Can you work these out from the model? Positions are in its coordinate system, mm. A direction names the side the tool comes from. Coordinates: 2 decimals unless noted, no trailing zeros. Order: outer loops, then holes, each group sorted by start corner. A loop starts at its lowest first (then second) coordinate and runs counter-clockwise, first axis right, second up. Notation, with made-up numbers: (-13, 87) -> (34, 87) arc R22 ccw to (34, 97) -> close; hole circle Ø7 at (-27.75, -11). An arc over 180 degrees is marked (long way). Return JSON: item names as keys, results as strings. Group by question number.
1) For faces 4 (the flat face through (0, 2, -11)), 5 (the flat face through (4, 2, -147.6)), 6 (the flat face through (23.435, 2, -150)), 7 (the flat face through (-20.58, 2, -48)), 8 (the flat face through (35, 4.8, -77)), which set-ups out of +Z, -Z, +X, -X, +Y, -Y let a thin tool reach every point of the face, with its end or its side?
2) If we section it at A-A, the plane z = -25.95: Please give me the cut outline in (x, y).
3) Thinking about a two-plate mould opening in X: for faces 1 (the cylindrical face through (-6.69, 2.43, -72.65)), 2 (the flat face through (12, 2, -152.4)), 3 (the flat face through (96.655, 2, -75)), which applies, +X half, -X half, draft (parallel to the pull), parting line (faces both ways), or undercut?
4) For pin 1 (2.5 mm diameter, centred on y = 2, z = -150, fed in from -X), with a flat end and sliding along its axis, tell me the tip position at first contact or that it passes through.
5) If we section it at B-B, the plane x = 33.5: Please give me the cut outline in (y, z), then the cut area to 3 significant figures.
6) If I drill on probe 1 along Z at (x, y) = (4.5, 0.55); probe 2 along X at (y, z) = (1.65, -25.95); probe 3 along Z at (x, y) = (11, 3.85), over which ranges is the centre line in solid material (lowest first)? Write a range as from..to.
7) If we section it at C-C, the plane y = 3.6: State how many separate pieces and enclosed holes the cut face has, then the cut area to 3 significant figures.
from build123d import *

# Parameters (mm, degrees)
SKETCH1_W           = 96.655493252
SKETCH1_H           = 152.4
BOSS_EXTRUDE1_DEPTH = 4.800000052
SKETCH3_W           = 7.8117192
SKETCH3_H           = 4.800000052
CUT_EXTRUDE2_DEPTH  = 181.530009628
SKETCH5_W           = 8.5
SKETCH5_H           = 2.852224977
CUT_EXTRUDE3_DEPTH  = 181.530009628
SKETCH6_W           = 101.6
SKETCH6_H           = 4.800000052
BOSS_EXTRUDE2_DEPTH = 25.4
SKETCH7_R           = 3.683
CUT_EXTRUDE4_DEPTH  = 181.530009628
SKETCH8_W           = 8.466666666
SKETCH8_H           = 4.826
SKETCH8_W_2         = 8.466666667
CUT_EXTRUDE5_DEPTH  = 181.530009628
SKETCH9_R           = 1.00000054
SKETCH9_R_2         = 1
SKETCH9_R_3         = 1.016
SKETCH9_R_4         = 4.899999979
CUT_EXTRUDE6_DEPTH  = 181.530009628


with BuildPart() as part:
    # Sketch1 → Boss-Extrude1 (new body)
    with BuildSketch(Plane(origin=(0, 0, 0), x_dir=(1, 0, 0), z_dir=(0, 1, 0))):
        with Locations((48.327746626, 76.2)):
            Rectangle(SKETCH1_W, SKETCH1_H)
    extrude(amount=BOSS_EXTRUDE1_DEPTH)

    # Sketch3 → Cut-Extrude2 (cut, through all)
    with BuildSketch(Plane.XZ):
        with Locations((3.9058596, -149.999999974)):
            Rectangle(SKETCH3_W, SKETCH3_H)
        with Locations((19.529298, -149.999999974)):
            Rectangle(SKETCH3_W, SKETCH3_H)
        with Locations((35.1527364, -149.999999974)):
            Rectangle(SKETCH3_W, SKETCH3_H)
        with Locations((27.3410172, -37.473737167)):
            Rectangle(SKETCH3_W, SKETCH3_H)
        with Locations((11.655298, -37.473737167)):
            Rectangle(SKETCH3_W, SKETCH3_H)
        with Locations((11.655298, -15.608000026)):
            Rectangle(SKETCH3_W, SKETCH3_H)
        with Locations((27.3410172, -15.608000026)):
            Rectangle(SKETCH3_W, SKETCH3_H)
    extrude(amount=-CUT_EXTRUDE2_DEPTH, mode=Mode.SUBTRACT)

    # Sketch5 → Cut-Extrude3 (cut, through all)
    with BuildSketch(Plane(origin=(0, 0, 0), x_dir=(-1, 0, 0), z_dir=(0, -1, 0))):
        with Locations((-20.288559041, 32.636660711)):
            Rectangle(SKETCH5_W, SKETCH5_H)
    extrude(amount=-CUT_EXTRUDE3_DEPTH, mode=Mode.SUBTRACT)

    # Sketch6 → Boss-Extrude2 (add)
    with BuildSketch(Plane.ZY):
        with Locations((-73.799999974, 2.400000026)):
            Rectangle(SKETCH6_W, SKETCH6_H)
    extrude(amount=BOSS_EXTRUDE2_DEPTH)

    # Sketch7 → Cut-Extrude4 (cut, through all)
    with BuildSketch(Plane(origin=(0, 4.800000052, 0), x_dir=(1, 0, 0), z_dir=(0, 1, 0))):
        with Locations(Location((-7.800402362, 76.161515735, 0), (0, 0, 270))):
            Circle(SKETCH7_R)
    extrude(amount=-CUT_EXTRUDE4_DEPTH, mode=Mode.SUBTRACT)

    # Sketch8 → Cut-Extrude5 (cut, through all)
    with BuildSketch(Plane(origin=(0, 4.800000052, 0), x_dir=(1, 0, 0), z_dir=(0, 1, 0))):
        with Locations((-16.346648987, 48.284809597)):
            Rectangle(SKETCH8_W, SKETCH8_H)
        with Locations((0.586684347, 48.284809597)):
            Rectangle(SKETCH8_W_2, SKETCH8_H)
        with Locations((-16.346648987, 104.21722165)):
            Rectangle(SKETCH8_W, SKETCH8_H)
        with Locations((0.586684347, 104.21722165)):
            Rectangle(SKETCH8_W_2, SKETCH8_H)
    extrude(amount=-CUT_EXTRUDE5_DEPTH, mode=Mode.SUBTRACT)

    # Sketch9 → Cut-Extrude6 (cut, through all)
    with BuildSketch(Plane(origin=(0, 4.800000052, 0), x_dir=(1, 0, 0), z_dir=(0, 1, 0))):
        with Locations(Location((71.255493252, 118.448957867, 0), (0, 0, 270))):
            Circle(SKETCH9_R)
        with Locations(Location((71.255493252, 134.448957871, 0), (0, 0, 270))):
            Circle(SKETCH9_R_2)
        with Locations(Location((71.713159771, 33.950000045, 0), (0, 0, 270))):
            Circle(SKETCH9_R_3)
        with Locations(Location((71.713159771, 17.950000041, 0), (0, 0, 270))):
            Circle(SKETCH9_R_3)
        with Locations(Location((71.713159771, 25.950000043, 0), (0, 0, 270))):
            Circle(SKETCH9_R_4)
        with Locations(Location((71.255493252, 126.448957869, 0), (0, 0, 270))):
            Circle(SKETCH9_R_4)
    extrude(amount=-CUT_EXTRUDE6_DEPTH, mode=Mode.SUBTRACT)


solid = part.part
Result sheet:
{
 "1": {"face 4": "+Z, -X, +Y, -Y", "face 5": "-Z, -X, +Y, -Y", "face 6": "-Z, +Y, -Y", "face 7": "+Y, -Y", "face 8": "+Z, -Z, +X, -X, +Y"},
 "2": {"outline": "(-25.4, 0) -> (66.81, 0) -> (66.81, 4.8) -> (-25.4, 4.8) -> close; (76.61, 0) -> (96.66, 0) -> (96.66, 4.8) -> (76.61, 4.8) -> close"},
 "3": {"face 1": "undercut", "face 2": "draft", "face 3": "+X half"},
 "4": {"pin 1": "stops at x = 7.81"},
 "5": {"outline": "(0, -147.6) -> (4.8, -147.6) -> (4.8, 0) -> (0, 0) -> close", "area": "708 mm2"},
 "6": {"probe 1": "z = -147.6..-106.63, -101.8..-50.7, -45.87..0", "probe 2": "x = -25.4..66.81, 76.61..96.66", "probe 3": "z = -152.4..-39.87, -35.07..-18.01, -13.21..0"},
 "7": {"separate pieces": "1", "enclosed holes": "16", "area": "16,700 mm2"}
}
